Input: part model. Units: mm. Frame: model coordinates. A direction names the side the tool comes from. Coordinates: 2 decimals unless noted, no trailing zeros. Loops run counter-clockwise (first coordinate to the right, second up) from the corner with the lowest first, then second, coordinate; pieces in that order, holes last.
Item 1: Reachability of faces 1 (the flat face through (-23, 0, 20)), 2 (the cylindrical face through (8.84, -1.8, 1.25)), 3 (the cylindrical face through (24.687, 5.978, 20.183)) from +Z, -Z, +X, -X, +Y, -Y: full face, straight path, thin tool, end or side. Return the list, or none.
Item 2: Section C-C on z = 22. Return loops of the section in (x, y), and give its area (3 significant figures).
Item 3: Section A-A on x = 5. Return loops of the section in (y, z), and give its area (3 significant figures).
Item 4: Section D-D on y = -16.5. Return loops of the section in (x, z), and give its area (3 significant figures).
Item 5: Section B-B on y = -1. Return loops of the section in (x, z).
Item 6: Ray query, line 1 along X through (y, z) = (0.5, 18.5); line 2 along Y through (x, z) = (0, 24); line 3 along Y through (x, z) = (15.5, 3). Return the intervals inside material, ascending.
Item 7: Contact query for flat-ended pins moving along their axis: P1, Ø6, axis at y = 20.5, z = 29, coming from the -X side; P2, Ø2.5, axis at x = 9.779, y = 0, coming from the -Z side; P3, Ø1.5, axis at x = 1.5, z = 18.5, coming from the -Y side; P4, Ø6, axis at x = 23.5, z = 31.5, coming from the +Y side. Output: stop coordinate, or through.
Item 8: Pull-direction query (Y, two-part tool) for faces 4 (the cylindrical face through (6.745, -30.375, 1.252)), 5 (the flat face through (-21.15, -8.76, 20.18)), 6 (the flat face through (0.4, -6.5, 0)); classes: released by +Y, released by -Y, zero draft, split by the parting line, or undercut.
```python
from build123d import *

# Parameters (mm, degrees)
F0_W     = 5.08
F0_H     = 34.798
F1_ANGLE = 337.5
F3_R     = 2.032
F4_DEPTH = 10.60485


with BuildPart() as f1:
    # F0 (on Front) → F1 (revolve)
    with BuildSketch(Plane.XZ):
        with Locations((-22.86, 19.939)):
            Rectangle(F0_W, F0_H)
    revolve(axis=Axis((0, 0, 19.939), (0, 0, -1)), revolution_arc=F1_ANGLE)

    # F0 (on Front) → F2 (revolve)
    with BuildSketch(Plane.XZ):
        Polygon((-31.115, 0), (0, 0), (0, 2.54), (-20.32, 2.54), (-25.4, 2.54), (-31.115, 2.54), align=None)
    revolve(axis=Axis((0, 0, 19.939), (0, 0, -1)))

    # F3 (on face) → F4 (cut)
    with BuildSketch(Plane(origin=(0, 0, 0), x_dir=(1, 0, 0), z_dir=(0, 0, -1))):
        with BuildLine():
            Line((0, 0), (6.35, 0))
            ThreePointArc((6.35, 0), (4.490128, 4.490128), (0, 6.35))
            Line((0, 6.35), (0, 0))
        make_face()
        with BuildLine():
            ThreePointArc((2.032, -9.779), (1.436841, -8.342159), (0, -7.747))
            ThreePointArc((0, -7.747), (-1.436841, -11.215841), (2.032, -9.779))
        make_face()
        with Locations((-9.779, 0)):
            Circle(F3_R)
        with BuildLine():
            ThreePointArc((2.032, 9.779), (-1.436841, 11.215841), (0, 7.747))
            ThreePointArc((0, 7.747), (1.436841, 8.342159), (2.032, 9.779))
        make_face()
        with BuildLine():
            ThreePointArc((0, -6.35), (4.490128, -4.490128), (6.35, 0))
            Line((6.35, 0), (0, 0))
            Line((0, 0), (0, -6.35))
        make_face()
        with BuildLine():
            ThreePointArc((11.811, 0), (9.779, 2.032), (7.747, 0))
            ThreePointArc((7.747, 0), (9.779, -2.032), (11.811, 0))
        make_face()
        with BuildLine():
            Line((0, 0), (0, 6.35))
            ThreePointArc((0, 6.35), (-4.490128, 4.490128), (-6.35, 0))
            Line((-6.35, 0), (0, 0))
        make_face()
        with BuildLine():
            ThreePointArc((-6.35, 0), (-4.490128, -4.490128), (0, -6.35))
            Line((0, -6.35), (0, 0))
            Line((0, 0), (-6.35, 0))
        make_face()
    extrude(amount=-F4_DEPTH, mode=Mode.SUBTRACT)


solid = f1.part
```
Results found:
1. face 1: +Z, -X
1. face 2: +Z, -Z
1. face 3: +Z
2. outline: (-25.4, 0) - (-20.32, 0) arc R20.32 cw (long way) to (-18.77, -7.78) - (-23.47, -9.72) arc R25.4 ccw (long way) to start
2. area: 684 mm2
3. outline: (-30.71, 0) - (-3.91, 0) - (-3.91, 2.54) - (-19.7, 2.54) - (-19.7, 37.34) - (-24.9, 37.34) - (-24.9, 2.54) - (-30.71, 2.54) - close; (3.91, 0) - (30.71, 0) - (30.71, 2.54) - (24.9, 2.54) - (24.9, 37.34) - (19.7, 37.34) - (19.7, 2.54) - (3.91, 2.54) - close
3. area: 499 mm2
4. outline: (-26.38, 0) - (26.38, 0) - (26.38, 2.54) - (19.31, 2.54) - (19.31, 37.34) - (11.86, 37.34) - (11.86, 2.54) - (-11.86, 2.54) - (-11.86, 37.34) - (-19.31, 37.34) - (-19.31, 2.54) - (-26.38, 2.54) - close
4. area: 653 mm2
5. outline: (-31.1, 0) - (-11.55, 0) - (-11.55, 2.54) - (-31.1, 2.54) - close; (-8.01, 0) - (-6.27, 0) - (-6.27, 2.54) - (-8.01, 2.54) - close; (6.27, 0) - (8.01, 0) - (8.01, 2.54) - (6.27, 2.54) - close; (11.55, 0) - (31.1, 0) - (31.1, 2.54) - (25.38, 2.54) - (25.38, 37.34) - (20.3, 37.34) - (20.3, 2.54) - (11.55, 2.54) - close
6. line 1: x = -25.4 to -20.31, 20.31 to 25.4
6. line 2: y = -25.4 to -20.32, 20.32 to 25.4
6. line 3: y = -20.12 to -13.14, 13.14 to 20.12
7. P1: stops at x = -18.41
7. P2: passes through
7. P3: stops at y = -25.39
7. P4: stops at y = 15
8. face 4: split by the parting line
8. face 5: undercut
8. face 6: zero draft
